Check sheet for the drawn part. Datum: minimum x, y, z corner. Units: mm. A direction names the side the tool comes from. Round coordinates to 2 decimals unless told otherwise and drop trailing zeros. Write each loop counter-clockwise with the first axis right and the second up, starting at its lowest first coordinate (ties: lowest second). Pieces come first, ordered by that corner, then holes. Notation, with made-up numbers: (-38.5, -32) - (-9.5, -32) arc R8 ccw to (-9.5, -26) - close; hole circle Ø10 at (-1, -5). An arc over 180 degrees is marked (long way). Answer as a JSON object with one key per item and string values. Group by question number.
Item 1: Sectioned sample at B-B on y = 24. Record the boundary of the cut face in (x, z), plus the area to 3 significant figures.
Item 2: Set-up check for the marked faces 1 and 2: record each of +Z, -Z, +X, -X, +Y, -Y from which the full face is reachable in a straight line by a thin tool's end or side.
Item 3: Thickness scan on line 1 (Z direction, x = 17.5, y = 25). Record the ranges inside material, lowest first.
Item 4: Gauge pin test, flat ends, axial feed: P1, Ø8.5, axis at x = 8.5, z = 19, coming from the +Y side; P2, Ø6, axis at x = 19.5, y = 20, coming from the +Z side; P3, Ø1.5, axis at y = 3, z = 6.5, coming from the +X side. Record the tip position at first contact, or that the pin passes through.
Item 5: Sectioned sample at A-A on x = 20.25. Record the boundary of the cut face in (y, z), plus the area to 3 significant figures.
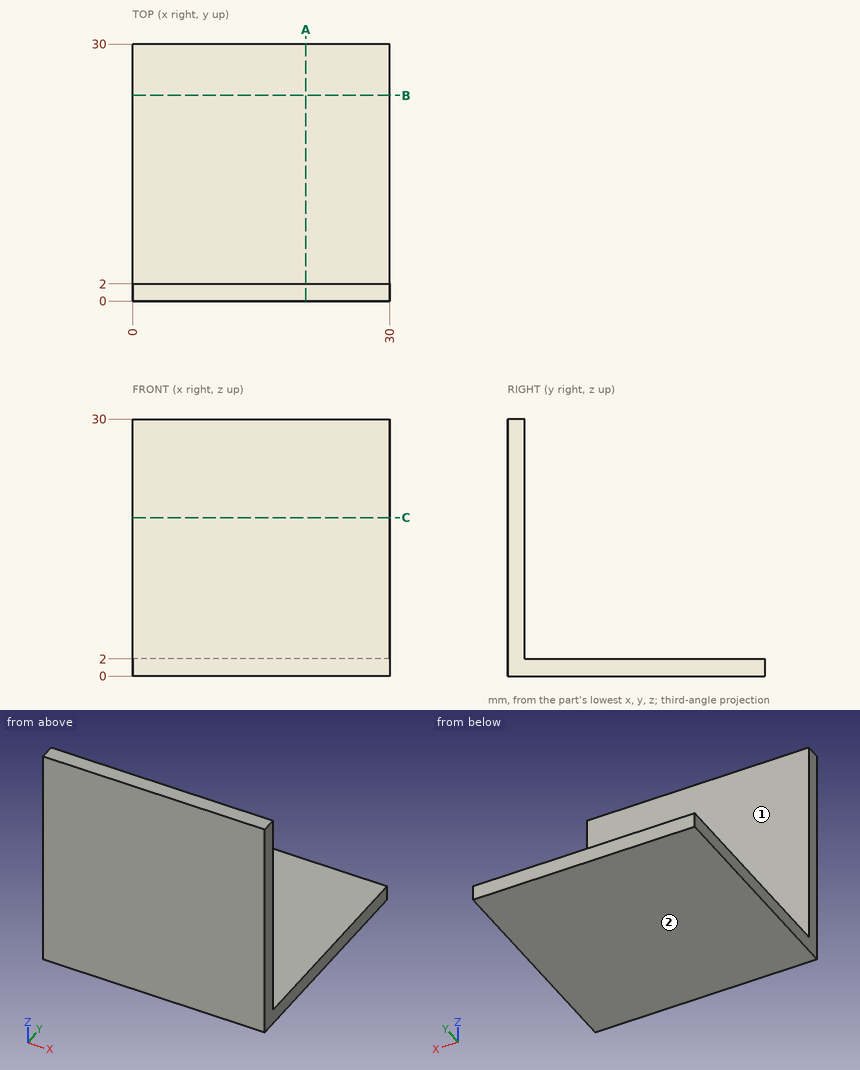
Completed:
{
 "1": {"outline": "(0, 0) - (30, 0) - (30, 2) - (0, 2) - close", "area": "60.0 mm²"},
 "2": {"face 1": "+Z, +X, -X, +Y", "face 2": "-Z, +X, -X, +Y, -Y"},
 "3": {"line 1": "0 to 2"},
 "4": {"P1": "y = 2", "P2": "z = 2", "P3": "through"},
 "5": {"outline": "(0, 0) - (30, 0) - (30, 2) - (2, 2) - (2, 30) - (0, 30) - close", "area": "116 mm²"}
}
